Part model, mm, in its own coordinate system. Face numbers are marked on the shaded views. Give positions to 0.01 mm unless a question says otherwise; leave off trailing zeros. Order: outer loops, then holes, each group sorted by start corner. A loop starts at its lowest first (then second) coordinate and runs counter-clockwise, first axis right, second up. Notation, with made-up numbers: (64.25, -27.75) - (76.25, -27.75) arc R30 ccw to (76.25, 10.25) - close; hole circle Ø3 at (53, 8). An arc over 180 degrees is marked (long way). Use one line per item in the form item = value. Start each with the question number.
1. Band-saw the part on A-A, the plane z = 139.5. List the corners of the cut face in (x, y), plus the area to 3 significant figures.
2. Pin check, flat tips, straight feed: P1, Ø1.5, axis at x = -39.5, y = 49.5, coming from the -Z side; P2, Ø8, axis at x = -31.5, z = 61.5, coming from the +Y side; P3, Ø4, axis at x = -37, y = 34.5, coming from the -Z side. Stop position of each tip, or through.
3. Drill centre lines: line 1 (Y direction, x = -39, z = 36); line 2 (Y direction, x = -50.5, z = 28.5); line 3 (X direction, y = 31, z = 36.5). Where is each one in solid material? Low to high.
4. Band-saw the part on C-C, the plane z = 161. List the corners of the cut face in (x, y).
5. Pull direction Y, two halves, no side cores. Call the marked faces 1 and 2: +Y half, -Y half, draft (parallel to the pull), parting line (faces both ways), or undercut.
6. Band-saw the part on B-B, the plane z = 36.5. List the corners of the cut face in (x, y).
from build123d import *

# Parameters (mm, degrees)
F0_R     = 50.8
F1_DEPTH = 189.992
F2_SIZE2 = 50.8
F2_SIZE  = 189.5881810245
F4_D     = 86.36
F4_DEPTH = 18.542
F4_TIP   = 25.9451615296


with BuildPart() as f1:
    # F0 (on Top) → F1 (new body)
    with BuildSketch(Plane.XY):
        with Locations((-50.3493994474, 45.8692982793)):
            Circle(F0_R)
    extrude(amount=F1_DEPTH)

    # F2
    f2_edges = [f1.edges().sort_by_distance(p)[0] for p in [
        (-101.149399, 45.869298, 189.992),
    ]]
    f2_side = f1.faces().sort_by_distance((-101.149399, 45.869298, 94.996))[0]
    chamfer(f2_edges, length=F2_SIZE, length2=F2_SIZE2, reference=f2_side)

    # F4
    with Locations(Plane(origin=(0, 0, 0), x_dir=(1, 0, 0), z_dir=(0, 0, -1))):
        with Locations((-47.8219240904, -45.9640063345)):
            Hole(F4_D / 2, depth=F4_DEPTH)
            with Locations((0, 0, -(F4_DEPTH + F4_TIP / 2))):  # 118° drill point
                Cone(0, F4_D / 2, F4_TIP, mode=Mode.SUBTRACT)


solid = f1.part
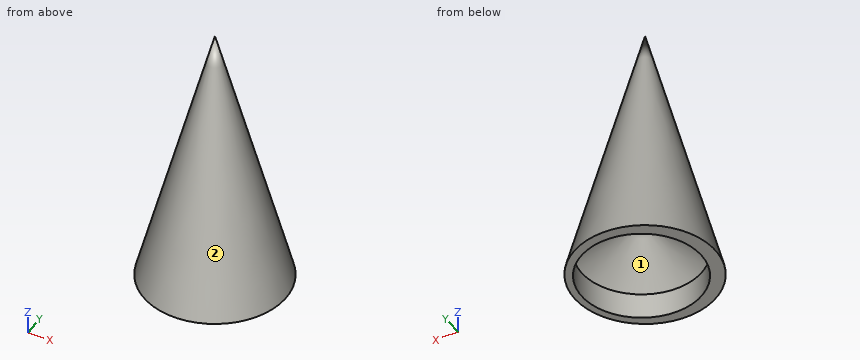
From the geometry:
q1.outline = circle Ø27.06 at (-50.35, 45.87)
q1.area = 575 mm²
q2.P1 = 38.6
q2.P2 = 77.27
q2.P3 = 33.81
q3.line_1 = 6.2 to 34.93, 57 to 85.54
q3.line_2 = 2.6 to 19.49, 72.44 to 89.14
q3.line_3 = -88.7 to -12
q4.outline = circle Ø15.54 at (-50.35, 45.87)
q5.face_1 = undercut
q5.face_2 = parting line
q6.outline = circle Ø82.26 at (-50.35, 45.87); hole circle Ø26.59 at (-47.82, 45.96)
